CAD build for the part. Positions are in the model's coordinates, mm. Face numbers are marked on the shaded views. A direction names the side the tool comes from. Round coordinates to 2 decimals unless told otherwise and drop trailing zeros. Write each loop counter-clockwise with the first axis right and the second up, starting at its lowest first coordinate (ties: lowest second). Pieces come first, ordered by that corner, then holes. Notation, with made-up numbers: (3, 86) - (30, 86) arc R22 ccw to (30, 113) - close; hole circle Ø2 at (44.5, -35). An arc over 180 degrees is marked (long way). Answer in a Markdown table with one row per item.
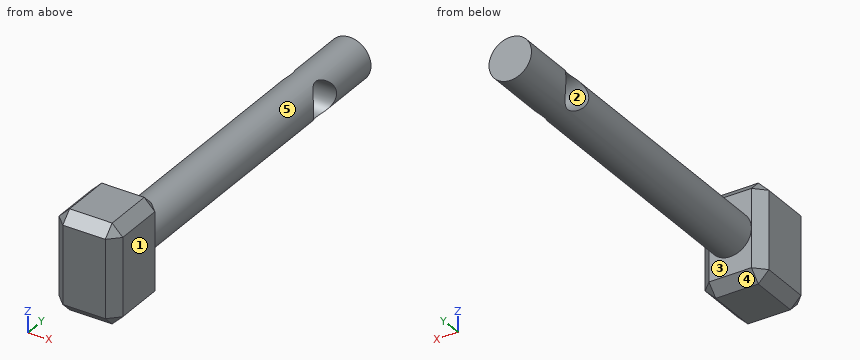
Autodesk Inventor part; units mm, degrees
ref_plane "工作平面1" through (0, 48, 0) normal (0, 1, 0) x (1, 0, 0)
ref_plane "YZ Plane" through (0, 0, 0) normal (1, 0, 0) x (0, 1, 0)
ref_plane "XZ Plane" through (0, 0, 0) normal (0, 1, 0) x (-1, 0, 0)
sketch "草圖1" plane through (0, 0, 0) normal (0, 0, 1) x (1, 0, 0)
  line L0 (0, 0) -> (3, 0)
  line L1 (3, 0) -> (3, 58)
  line L2 (3, 58) -> (0, 58)
  line L3 (0, 58) -> (0, 0)
  dimension "d0" = 58
  dimension "d1" = 3
revolve "迴轉1" add sketch "草圖1" angle 360 about axis through (0, 58, 0) along (0, -1, 0)
ref_plane "工作平面1" through (0, 48, 0) normal (0, 1, 0) x (1, 0, 0)
sketch "草圖2" plane through (0, 48, 0) normal (0, 1, 0) x (1, 0, 0)
  line L0 (-10.3022, 0) -> (10.735, 0)
  line L1 (10.735, 0) -> (10.735, 2.5)
  line L2 (10.735, 2.5) -> (-10.3022, 2.5)
  line L3 (-10.3022, 2.5) -> (-10.3022, 0)
  point P0 (0, 0)
  dimension "d4" = 2.5
  dimension "d5" = 0
revolve "迴轉2" cut sketch "草圖2" angle 360 about axis through (-10.3022, 48, 0) along (1, 0, 0)
sketch "草圖3" plane through (0, 0, 0) normal (0, -1, 0) x (1, 0, 0)
  line L0 (-4.5, 7) -> (4.5, 7)
  line L1 (4.5, 7) -> (4.5, -7)
  line L2 (4.5, -7) -> (-4.5, -7)
  line L3 (-4.5, -7) -> (-4.5, 7)
  point P0 (0, 0)
  dimension "d7" = 9
  dimension "d8" = 4.5
  dimension "d9" = 14
  dimension "d10" = 7
extrude "擠出1" add sketch "草圖3" against normal blind 10
chamfer "倒角1" distance 1.5 angle 45 12 edges at (4.5, 5, -7) (4.5, 5, 7) (-4.5, 5, 7) (-4.5, 5, -7) (0, 0, -7) (-4.5, 0, 0) (4.5, 0, 0) (0, 0, 7) (0, 10, -7) (4.5, 10, 0) (0, 10, 7) (-4.5, 10, 0)
properties part number "槌子"
Q1. Drill centre lines: line 1 (Y direction, x = 0.75, z = 0); line 2 (Z direction, x = 0.25, y = 48); line 3 (Y direction, x = -1, z = -4.25). Where is each one in solid material? Low to high.
Computed:
| item | result |
|---|---|
| line 1 | y = 0 to 45.5, 50.5 to 58 |
| line 2 | z = -2.99 to -2.5, 2.5 to 2.99 |
| line 3 | y = 0 to 10 |
Q2. Saw through at A-A on z = -1.25. List the corners of the cut face in (x, y), then the cut area to 3 significant figures.
Computed:
| item | result |
|---|---|
| outline | (-4.5, 1.5) - (-3, 0) - (3, 0) - (4.5, 1.5) - (4.5, 8.5) - (3, 10) - (2.73, 10) - (2.73, 45.83) - (-2.73, 45.83) - (-2.73, 10) - (-3, 10) - (-4.5, 8.5) - close; (-2.73, 50.17) - (2.73, 50.17) - (2.73, 58) - (-2.73, 58) - close |
| area | 324 mm2 |
Q3. Pull direction Y, two halves, no side cores. Call the marked faces 1, 2 and 3: released by +Y, released by -Y, zero draft, split by the parting line, or undercut.
Computed:
| item | result |
|---|---|
| face 1 | zero draft |
| face 2 | undercut |
| face 3 | released by +Y |
Q4. Saw through at C-C on x = 2.5. List the corners of the cut face in (y, z).
Computed:
| item | result |
|---|---|
| outline | (0, -5.5) - (1.5, -7) - (8.5, -7) - (10, -5.5) - (10, -1.66) - (46.13, -1.66) arc R2.5 cw to (46.13, 1.66) - (10, 1.66) - (10, 5.5) - (8.5, 7) - (1.5, 7) - (0, 5.5) - close; (49.87, -1.66) - (58, -1.66) - (58, 1.66) - (49.87, 1.66) arc R2.5 cw to start |
Q5. Saw through at B-B on x = 0. List the corners of the cut face in (y, z).
Computed:
| item | result |
|---|---|
| outline | (0, -5.5) - (1.5, -7) - (8.5, -7) - (10, -5.5) - (10, -3) - (58, -3) - (58, 3) - (10, 3) - (10, 5.5) - (8.5, 7) - (1.5, 7) - (0, 5.5) - close; hole circle Ø5 at (48, 0) |
Q6. Saw through at D-D on y = 53.5. List the corners of the cut face in (x, z).
Computed:
| item | result |
|---|---|
| outline | circle Ø6 at (0, 0) |
Q7. 3-axis set-ups, long thin cutter, end or side, ignore diameter. For the marked faces 4 and 5: which of +Z, -Z, +X, -X, +Y, -Y reach the whole face in a straight line?
Computed:
| item | result |
|---|---|
| face 4 | -Z, +X, -X, +Y |
| face 5 | +Y |
Q8. Flat gauge pins, fed straight in: pin 1 (6 mm diameter, centred on y = 25, z = -2.5, fed in from +X); pin 2 (3 mm diameter, centred on y = 44, z = 2.5, fed in from +X); pin 3 (6 mm diameter, centred on y = 41.5, z = -5.5, fed in from +X). Where does each tip first touch, or does it go through?
Computed:
| item | result |
|---|---|
| pin 1 | stops at x = 3 |
| pin 2 | stops at x = 2.83 |
| pin 3 | stops at x = 1.66 |
